Can you work these out from the model? Positions are in its coordinate system, mm. Face numbers are marked on the shaded views. Coordinates: 2 decimals unless noted, no trailing zeros. Order: outer loops, then holes, each group sorted by start corner. A loop starts at its lowest first (then second) coordinate and runs counter-clockwise, first axis right, second up. Notation, with made-up numbers: (79.25, -11.75) -> (111.25, -11.75) arc R15 cw to (111.25, -7.75) -> close; hole circle Ø2 at (14.25, -5). An arc over 180 degrees is marked (long way). Answer in a Markdown table with one row per item.
```python
from build123d import *

# Parameters (mm, degrees)
F0_W     = 120
F0_H     = 240
F0_R     = 2
F0_R_2   = 22
F1_DEPTH = 15
F0_R_3   = 16.5
F2_DEPTH = 12
F0_R_4   = 1.75
F0_W_2   = 75
F0_H_2   = 95
F3_DEPTH = 13


# Not quite as in the source:
# - a feature names something its author has since deleted; it is built from what else it names


with BuildPart() as f1:
    # F0 (on Right) → F1 (new body)
    with BuildSketch(Plane.YZ):
        with Locations((-10.4347826087, 0)):
            Rectangle(F0_W, F0_H)
        with Locations((-60.4347826087, -112)):
            Circle(F0_R, mode=Mode.SUBTRACT)
        with Locations((39.5652173913, -112)):
            Circle(F0_R, mode=Mode.SUBTRACT)
        Polygon((-60.4347826087, -102.5), (-60.4347826087, 25.4482906163), (-60.4347826087, 34.5), (39.5652173913, 34.5), (39.5652173913, 25.4482906163), (39.5652173913, -102.5), align=None, mode=Mode.SUBTRACT)
        with Locations((-60.4347826087, 112)):
            Circle(F0_R, mode=Mode.SUBTRACT)
        with Locations((-10.4347826087, 78)):
            Circle(F0_R_2, mode=Mode.SUBTRACT)
        with Locations((39.5652173913, 112.0000034571)):
            Circle(F0_R, mode=Mode.SUBTRACT)
    extrude(amount=F1_DEPTH)

    # F0 (on Right) → F2 (join)
    with BuildSketch(Plane.YZ):
        with Locations((-10.4347826087, 78)):
            Circle(F0_R_2)
        with Locations((-10.4347826087, 78)):
            Circle(F0_R_3, mode=Mode.SUBTRACT)
    extrude(amount=F2_DEPTH)

    # F0 (on Right) → F3 (join)
    with BuildSketch(Plane.YZ):
        Polygon((-60.4347826087, 34.5), (-60.4347826087, 25.4482906163), (-60.4347826087, -102.5), (39.5652173913, -102.5), (39.5652173913, 25.4482906163), (39.5652173913, 34.5), align=None)
        with Locations((-53.4347826087, -93.5)):
            Circle(F0_R_4, mode=Mode.SUBTRACT)
        with Locations((32.5652173913, -93.5)):
            Circle(F0_R_4, mode=Mode.SUBTRACT)
        with Locations((-10.4347826087, -34)):
            Rectangle(F0_W_2, F0_H_2, mode=Mode.SUBTRACT)
        with Locations((-53.4347826087, 25.5)):
            Circle(F0_R_4, mode=Mode.SUBTRACT)
        with Locations((32.5652173913, 25.5)):
            Circle(F0_R_4, mode=Mode.SUBTRACT)
    extrude(amount=F3_DEPTH)


solid = f1.part
```
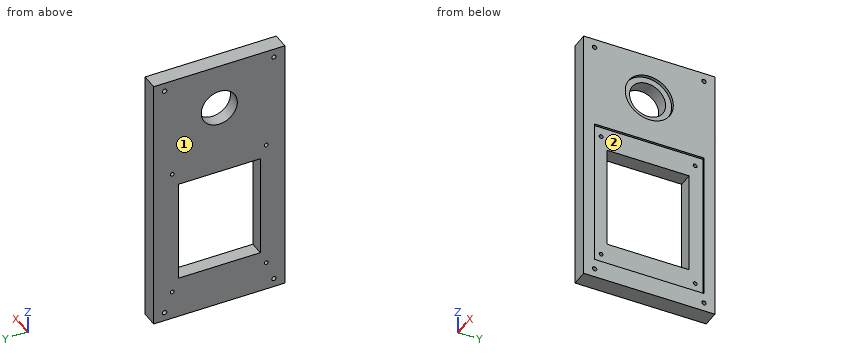
(1) Will this pin go through, and if not, where does the flat tip stop? pin 1 Ø5.5 at (y, z) = (-53.43, 25.5) entering from +X.
Response values:
| item | result |
|---|---|
| pin 1 | x = 13 |
(2) I need wall thicknesses on line 1 (Y direction, x = 8.5, z = -93.5); line 2 (Z direction, x = 4.25, y = -47); line 3 (Z direction, x = 4, y = -61). Which ranges of each line are inside material? Lowest first, please. Write a range as [from, to].
Response values:
| item | result |
|---|---|
| line 1 | [-70.43, -55.18], [-51.68, 30.82], [34.32, 49.57] |
| line 2 | [-120, -81.5], [13.5, 120] |
| line 3 | [-120, -113.92], [-110.08, 110.08], [113.92, 120] |
(3) Suppose I cut it at A-A (z = 10.5). Please give me the cut outline in (x, y).
Response values:
| item | result |
|---|---|
| outline | (0, -70.43) -> (15, -70.43) -> (15, -60.43) -> (13, -60.43) -> (13, -47.93) -> (0, -47.93) -> close; (0, 27.07) -> (13, 27.07) -> (13, 39.57) -> (15, 39.57) -> (15, 49.57) -> (0, 49.57) -> close |
(4) Suppose I cut it at B-B (x = 3.5). Count the separate pieces of the cut face and the enclosed holes in it, and give its area (3 significant figures).
Response values:
| item | result |
|---|---|
| separate pieces | 1 |
| enclosed holes | 10 |
| area | 20,700 mm2 |
(5) We'd pull the mould along Z, two halves only. Please class the marked faces 1 and 2: +Z half, -Z half, draft (parallel to the pull), parting line (faces both ways), or undercut.
Response values:
| item | result |
|---|---|
| face 1 | draft |
| face 2 | undercut |
